Source: CAD feature listing. Evaluate the final solid. Frame: model axes, mm. Round coordinates to 2 decimals unless told otherwise and drop trailing zeros. Write each loop counter-clockwise with the first axis right and the second up, starting at its lowest first coordinate (ties: lowest second). Pieces come first, ordered by that corner, then holes. Notation, with made-up numbers: (54.25, 54.25) -> (103.25, 54.25) arc R27 ccw to (103.25, 89.25) -> close; hole circle Ø8 at (37, 54.5). An arc over 180 degrees is marked (long way). Put each result on its own line as item: value.
```python
from build123d import *

# Parameters (mm, degrees)
SKETCH_W  = 60
SKETCH_H  = 80
PAD_DEPTH = 2


with BuildPart() as part:
    # Sketch → Pad (new body)
    with BuildSketch(Plane.XY.offset(32)):
        Rectangle(SKETCH_W, SKETCH_H)
        with BuildLine():
            ThreePointArc((1.623618, 5.270955), (0, 15), (-1.623618, 5.270955))
            Line((-1.623618, -24.016518), (-1.623618, 5.270955))
            Line((1.623618, -24.016518), (-1.623618, -24.016518))
            Line((1.623618, 5.270955), (1.623618, -24.016518))
        make_face(mode=Mode.SUBTRACT)
    extrude(amount=PAD_DEPTH)


solid = part.part
```
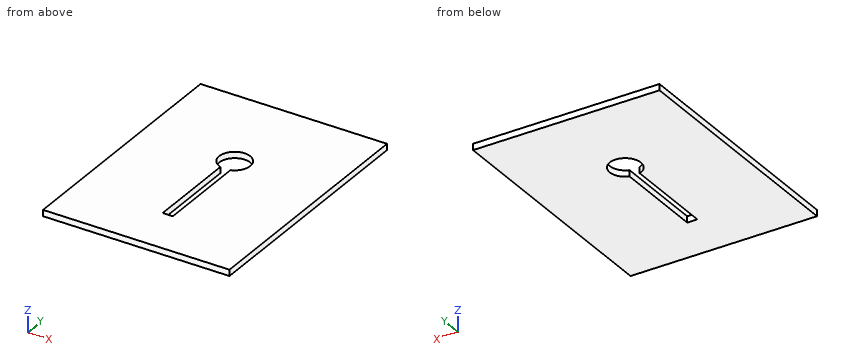
Q1. Cut plane B-B on y = -23. Output: boundary loops of the cut face in (x, z), and give its area (3 significant figures).
Ans:
outline: (-30, 32) -> (-1.62, 32) -> (-1.62, 34) -> (-30, 34) -> close; (1.62, 32) -> (30, 32) -> (30, 34) -> (1.62, 34) -> close
area: 114 mm^2
Q2. Material intervals for line 1 (Y direction, x = 0, z = 32.5); line 2 (X direction, y = -19, z = 33.35); line 3 (X direction, y = 10, z = 32.7), sorted ascending. Write a range as [from, to].
Ans:
line 1: y = [-40, -24.02], [15, 40]
line 2: x = [-30, -1.62], [1.62, 30]
line 3: x = [-30, -5], [5, 30]
Q3. Cut plane A-A on x = 0. Output: boundary loops of the cut face in (y, z).
Ans:
outline: (-40, 32) -> (-24.02, 32) -> (-24.02, 34) -> (-40, 34) -> close; (15, 32) -> (40, 32) -> (40, 34) -> (15, 34) -> close
Q4. Pin query (flat end, axial travel): pin 1 (9 mm diameter, centred on x = 0, y = 10, fed in from -Z). Return the tip coordinate at first contact, or that it passes through.
Ans:
pin 1: passes through
Q5. Cut plane C-C on z = 33. Output: boundary loops of the cut face in (x, y), and give its area (3 significant figures).
Ans:
outline: (-30, -40) -> (30, -40) -> (30, 40) -> (-30, 40) -> close; hole (-1.62, -24.02) -> (1.62, -24.02) -> (1.62, 5.27) arc R5 ccw (long way) to (-1.62, 5.27) -> close
area: 4,630 mm^2
